Here's the drawing with two shaded views (mm, measured from the low corner). I have some questions. Give positions to 0.01 mm unless a question says otherwise; leave off trailing zeros. Loops run counter-clockwise (first coordinate to the right, second up) from the corner with the lowest first, then second, coordinate; pieces in that order, holes last.
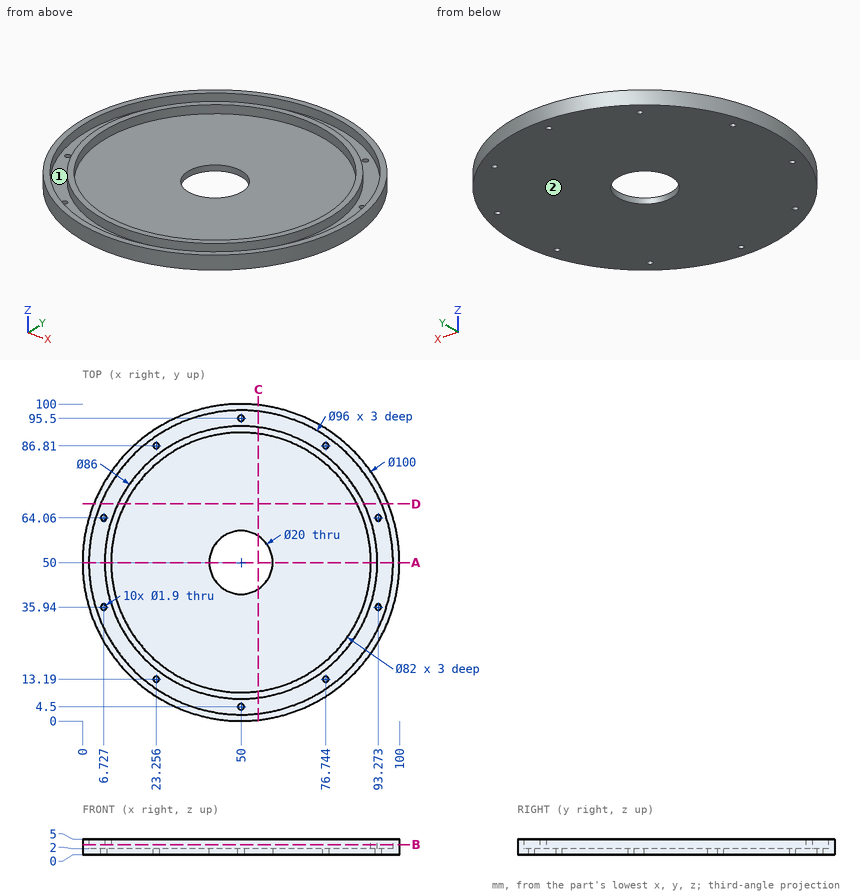
(1) Will these pins go through, and if not, where does the flat tip stop? P1, Ø1.5, axis at x = 50, y = 95.5, coming from the +Z side; P2, Ø2.5, axis at x = 93.27, y = 35.94, coming from the +Z side.
Returned:
P1: passes through
P2: stops at z = 2
(2) Suppose I cut it at D-D on y = 68.5. List the corners of the cut face in (x, z) for me, plus the area to 3 significant figures.
Returned:
outline: (3.55, 0) - (96.45, 0) - (96.45, 5) - (94.29, 5) - (94.29, 2) - (88.82, 2) - (88.82, 5) - (86.59, 5) - (86.59, 2) - (13.41, 2) - (13.41, 5) - (11.18, 5) - (11.18, 2) - (5.71, 2) - (5.71, 5) - (3.55, 5) - close
area: 212 mm2
(3) Suppose I cut it at C-C on x = 55.5. List the corners of the cut face in (y, z) for me.
Returned:
outline: (0.3, 0) - (41.65, 0) - (41.65, 2) - (9.37, 2) - (9.37, 5) - (7.35, 5) - (7.35, 2) - (2.32, 2) - (2.32, 5) - (0.3, 5) - close; (58.35, 0) - (99.7, 0) - (99.7, 5) - (97.68, 5) - (97.68, 2) - (92.65, 2) - (92.65, 5) - (90.63, 5) - (90.63, 2) - (58.35, 2) - close
(4) Suppose I cut it at B-B on z = 3.25. List the corners of the cut face in (x, y) for me, plus the area to 3 significant figures.
Returned:
outline: circle Ø100 at (50, 50); circle Ø86 at (50, 50); hole circle Ø96 at (50, 50); hole circle Ø82 at (50, 50)
area: 1,140 mm2
(5) Suppose I cut it at A-A on y = 50. List the corners of the cut face in (x, z) for me.
Returned:
outline: (0, 0) - (40, 0) - (40, 2) - (9, 2) - (9, 5) - (7, 5) - (7, 2) - (2, 2) - (2, 5) - (0, 5) - close; (60, 0) - (100, 0) - (100, 5) - (98, 5) - (98, 2) - (93, 2) - (93, 5) - (91, 5) - (91, 2) - (60, 2) - close
(6) Please list where these lines run through material, in increasing order: probe 1 along Y at (x, z) = (50, 0.8); probe 2 along Y at (x, z) = (50, 3.8); probe 3 along X at (y, z) = (64, 3.4) (1 decimal).
Returned:
probe 1: y = 0 to 3.55, 5.45 to 40, 60 to 94.55, 96.45 to 100
probe 2: y = 0 to 2, 7 to 9, 91 to 93, 98 to 100
probe 3: x = 2 to 4.1, 9.3 to 11.5, 88.5 to 90.7, 95.9 to 98
(7) Thinking about a two-plate mould opening in X: for the marked faces 1 and 2, which applies, pulls with the +X half, pulls with the -X half, needs draft (parallel to the pull), parting line crosses it, or undercut?
Returned:
face 1: undercut
face 2: needs draft
